Design review of the part built by this model. Coordinates are the model's own, in mm. Give positions to 0.01 mm unless a question says otherwise; leave off trailing zeros. Write each loop counter-clockwise with the first axis right and the second up, starting at its lowest first coordinate (ties: lowest second). Pieces come first, ordered by that corner, then holes. Notation, with made-up numbers: (17, 39.25) -> (41, 39.25) arc R25 cw to (41, 65.25) -> close; hole circle Ø3 at (12, 18.25). An arc over 180 degrees is marked (long way). Return JSON: item names as keys, results as strings. Group by question number.
from build123d import *

# Parameters (mm, degrees)
F0_W     = 76
F0_H     = 76
F1_DEPTH = 3
F3_DEPTH = 25
F4_R     = 3.75
F5_DEPTH = 25


with BuildPart() as f1:
    # F0 (on Top) → F1 (new body)
    with BuildSketch(Plane.XY):
        Rectangle(F0_W, F0_H)
    extrude(amount=F1_DEPTH)

    # F2 (on face) → F3 (cut)
    with BuildSketch(Plane.XY.offset(3)):
        with BuildLine():
            ThreePointArc((25.0727558965, 11.2963229308), (23.3008846492, 7.5709163622), (26.9240976399, 5.5984789253))
            ThreePointArc((26.9240976399, 5.5984789253), (26.1540541981, 8.4979673453), (25.0727558965, 11.2963229308))
        make_face()
        with BuildLine():
            ThreePointArc((25.0727558965, 11.2963229308), (26.1540541981, 8.4979673453), (26.9240976399, 5.5984789253))
            ThreePointArc((26.9240976399, 5.5984789253), (28.5320922892, 6.669051044), (29.1540541981, 8.4979673453))
            ThreePointArc((29.1540541981, 8.4979673453), (27.8505366022, 10.9722242949), (25.0727558965, 11.2963229308))
        make_face()
        with BuildLine():
            ThreePointArc((29.1540541981, -8.4979673453), (28.5320922892, -6.669051044), (26.9240976399, -5.5984789253))
            ThreePointArc((26.9240976399, -5.5984789253), (26.1540541981, -8.4979673453), (25.0727558965, -11.2963229308))
            ThreePointArc((25.0727558965, -11.2963229308), (27.8505366022, -10.9722242949), (29.1540541981, -8.4979673453))
        make_face()
        with BuildLine():
            ThreePointArc((25.0727558965, -11.2963229308), (26.1540541981, -8.4979673453), (26.9240976399, -5.5984789253))
            ThreePointArc((26.9240976399, -5.5984789253), (23.3008846492, -7.5709163622), (25.0727558965, -11.2963229308))
        make_face()
        with BuildLine():
            ThreePointArc((13.6444735922, 23.8763133752), (14.4007386812, 19.8209163622), (18.4913492013, 20.3548521172))
            ThreePointArc((18.4913492013, 20.3548521172), (16.164094438, 22.2479673453), (13.6444735922, 23.8763133752))
        make_face()
        with BuildLine():
            ThreePointArc((13.6444735922, 23.8763133752), (16.164094438, 22.2479673453), (18.4913492013, 20.3548521172))
            ThreePointArc((18.4913492013, 20.3548521172), (18.990909279, 21.2434187626), (19.164094438, 22.2479673453))
            ThreePointArc((19.164094438, 22.2479673453), (17.0129576374, 25.1253674337), (13.6444735922, 23.8763133752))
        make_face()
        with BuildLine():
            ThreePointArc((19.164094438, -22.2479673453), (18.990909279, -21.2434187626), (18.4913492013, -20.3548521172))
            ThreePointArc((18.4913492013, -20.3548521172), (16.164094438, -22.2479673453), (13.6444735922, -23.8763133752))
            ThreePointArc((13.6444735922, -23.8763133752), (17.0129576374, -25.1253674337), (19.164094438, -22.2479673453))
        make_face()
        with BuildLine():
            ThreePointArc((13.6444735922, -23.8763133752), (16.164094438, -22.2479673453), (18.4913492013, -20.3548521172))
            ThreePointArc((18.4913492013, -20.3548521172), (14.4007386812, -19.8209163622), (13.6444735922, -23.8763133752))
        make_face()
        with BuildLine():
            ThreePointArc((-2.9955338657, 27.3363636364), (0, 24.5), (2.9955338657, 27.3363636364))
            ThreePointArc((2.9955338657, 27.3363636364), (0, 27.5), (-2.9955338657, 27.3363636364))
        make_face()
        with BuildLine():
            ThreePointArc((-2.9955338657, 27.3363636364), (0, 27.5), (2.9955338657, 27.3363636364))
            ThreePointArc((2.9955338657, 27.3363636364), (2.9988832586, 27.4181513503), (3, 27.5))
            ThreePointArc((3, 27.5), (-0.0818486497, 30.4988832586), (-2.9955338657, 27.3363636364))
        make_face()
        with BuildLine():
            ThreePointArc((3, -27.5), (2.9988832586, -27.4181513503), (2.9955338657, -27.3363636364))
            ThreePointArc((2.9955338657, -27.3363636364), (0, -27.5), (-2.9955338657, -27.3363636364))
            ThreePointArc((-2.9955338657, -27.3363636364), (-0.0818486497, -30.4988832586), (3, -27.5))
        make_face()
        with BuildLine():
            ThreePointArc((-2.9955338657, -27.3363636364), (0, -27.5), (2.9955338657, -27.3363636364))
            ThreePointArc((2.9955338657, -27.3363636364), (0, -24.5), (-2.9955338657, -27.3363636364))
        make_face()
        with BuildLine():
            ThreePointArc((-13.164094438, 22.2479673453), (-13.2866943496, 23.0968305447), (-13.6444735922, 23.8763133752))
            ThreePointArc((-13.6444735922, 23.8763133752), (-16.164094438, 22.2479673453), (-18.4913492013, 20.3548521172))
            ThreePointArc((-18.4913492013, 20.3548521172), (-15.1595458553, 19.4211525044), (-13.164094438, 22.2479673453))
        make_face()
        with BuildLine():
            ThreePointArc((-18.4913492013, 20.3548521172), (-16.164094438, 22.2479673453), (-13.6444735922, 23.8763133752))
            ThreePointArc((-13.6444735922, 23.8763133752), (-17.9274501949, 24.6750183284), (-18.4913492013, 20.3548521172))
        make_face()
        with BuildLine():
            ThreePointArc((-18.4913492013, -20.3548521172), (-17.9274501949, -24.6750183284), (-13.6444735922, -23.8763133752))
            ThreePointArc((-13.6444735922, -23.8763133752), (-16.164094438, -22.2479673453), (-18.4913492013, -20.3548521172))
        make_face()
        with BuildLine():
            ThreePointArc((-18.4913492013, -20.3548521172), (-16.164094438, -22.2479673453), (-13.6444735922, -23.8763133752))
            ThreePointArc((-13.6444735922, -23.8763133752), (-13.2866943496, -23.0968305447), (-13.164094438, -22.2479673453))
            ThreePointArc((-13.164094438, -22.2479673453), (-15.1595458553, -19.4211525044), (-18.4913492013, -20.3548521172))
        make_face()
        with BuildLine():
            ThreePointArc((-23.1540541981, 8.4979673453), (-23.6797972485, 10.1944497494), (-25.0727558965, 11.2963229308))
            ThreePointArc((-25.0727558965, 11.2963229308), (-26.1540541981, 8.4979673453), (-26.9240976399, 5.5984789253))
            ThreePointArc((-26.9240976399, 5.5984789253), (-24.3251378968, 6.1199292542), (-23.1540541981, 8.4979673453))
        make_face()
        with BuildLine():
            ThreePointArc((-26.9240976399, 5.5984789253), (-26.1540541981, 8.4979673453), (-25.0727558965, 11.2963229308))
            ThreePointArc((-25.0727558965, 11.2963229308), (-29.007223747, 9.4250183284), (-26.9240976399, 5.5984789253))
        make_face()
        with BuildLine():
            ThreePointArc((-26.9240976399, -5.5984789253), (-29.007223747, -9.4250183284), (-25.0727558965, -11.2963229308))
            ThreePointArc((-25.0727558965, -11.2963229308), (-26.1540541981, -8.4979673453), (-26.9240976399, -5.5984789253))
        make_face()
        with BuildLine():
            ThreePointArc((-26.9240976399, -5.5984789253), (-26.1540541981, -8.4979673453), (-25.0727558965, -11.2963229308))
            ThreePointArc((-25.0727558965, -11.2963229308), (-23.6797972485, -10.1944497494), (-23.1540541981, -8.4979673453))
            ThreePointArc((-23.1540541981, -8.4979673453), (-24.3251378968, -6.1199292542), (-26.9240976399, -5.5984789253))
        make_face()
    extrude(amount=-F3_DEPTH, mode=Mode.SUBTRACT)

    # F4 (on face) → F5 (cut)
    with BuildSketch(Plane.XY.offset(3)):
        with Locations((-29.5, 29.5)):
            Circle(F4_R)
    extrude(amount=-F5_DEPTH, mode=Mode.SUBTRACT)


solid = f1.part
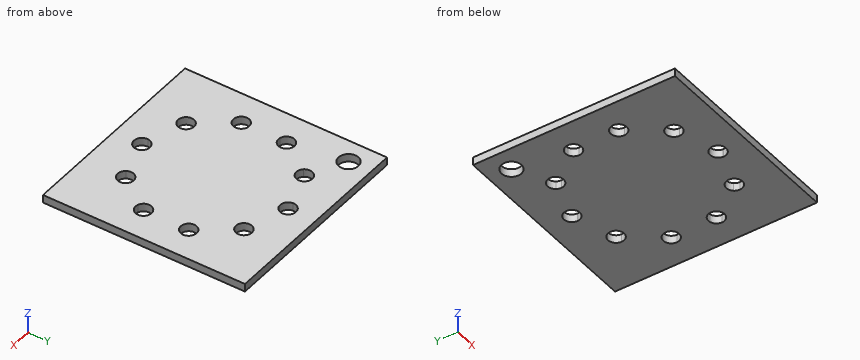
Q1. Take a section at A-A, the plane x = 0. Give the boundary of the cut face in (y, z).
Q2. Take a section at C-C, the plane x = -30.5. Give the boundary of the cut face in (y, z).
Q3. Take a section at D-D, the plane z = 1.85. Count the separate pieces of the cut face and the enclosed holes in it, plus the area to 3 significant figures.
Q4. For L1, parallel to Y at x = 17, z = 1.65; L2, parallel to Y at x = -29.5, z = 1.2; L3, parallel to Y at x = 1, z = 0.75, list the stretches that pass through material, from the lowest coordinate up. Write a range as from..to.
Q5. Take a section at B-B, the plane y = 29.5. Give the boundary of the cut face in (x, z).
Final values:
{
 "1": {"outline": "(-38, 0) -> (-30.5, 0) -> (-30.5, 3) -> (-38, 3) -> close; (-24.5, 0) -> (24.5, 0) -> (24.5, 3) -> (-24.5, 3) -> close; (30.5, 0) -> (38, 0) -> (38, 3) -> (30.5, 3) -> close"},
 "2": {"outline": "(-38, 0) -> (25.89, 0) -> (25.89, 3) -> (-38, 3) -> close; (33.11, 0) -> (38, 0) -> (38, 3) -> (33.11, 3) -> close"},
 "3": {"separate pieces": "1", "enclosed holes": "11", "area": "5,450 mm²"},
 "4": {"L1": "y = -38..-25.13, -19.37..19.37, 25.13..38", "L2": "y = -38..25.75, 33.25..38", "L3": "y = -38..-30.33, -24.67..24.67, 30.33..38"},
 "5": {"outline": "(-38, 0) -> (-33.25, 0) -> (-33.25, 3) -> (-38, 3) -> close; (-25.75, 0) -> (-2.24, 0) -> (-2.24, 3) -> (-25.75, 3) -> close; (2.24, 0) -> (38, 0) -> (38, 3) -> (2.24, 3) -> close"}
}
